Build history of the part. All positions in model axes, mm. Round coordinates to 2 decimals unless told otherwise and drop trailing zeros. Order: outer loops, then holes, each group sorted by start corner. A loop starts at its lowest first (then second) coordinate and runs counter-clockwise, first axis right, second up. Notation, with made-up numbers: M 65.5,85 L 75.5,85 A21 ccw 75.5,117 Z; hole C 80,-0.5 d2. An arc over 180 degrees is marked long. Use CSV: the item, a comma, the result in double quotes.
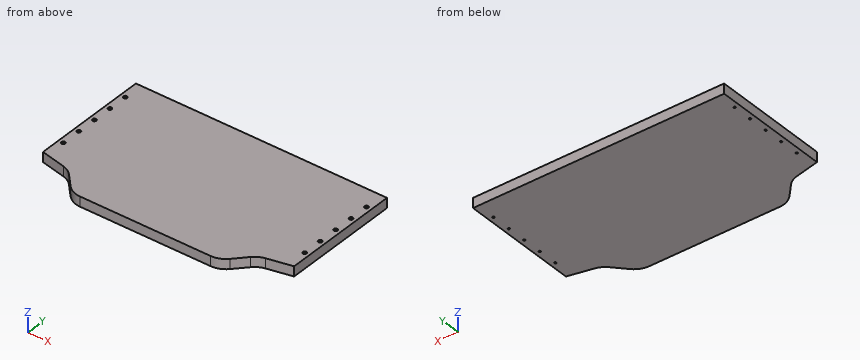
from build123d import *

# Parameters (mm, degrees)
BOSS_EXTRUDE1_DEPTH                        = 25.4
FILLET1_R                                  = 50.8
CSK_FOR_10_FLAT_HEAD_MACHINE_SCREW_2_COUNT = 2
CSK_FOR_10_FLAT_HEAD_MACHINE_SCREW_2_PITCH = 50.8
CSK_FOR_10_FLAT_HEAD_MACHINE_SCREW_3_COUNT = 2
CSK_FOR_10_FLAT_HEAD_MACHINE_SCREW_3_PITCH = 101.6
CSK_FOR_10_FLAT_HEAD_MACHINE_SCREW_4_COUNT = 2
CSK_FOR_10_FLAT_HEAD_MACHINE_SCREW_4_PITCH = 152.4
CSK_FOR_10_FLAT_HEAD_MACHINE_SCREW_5_COUNT = 2
CSK_FOR_10_FLAT_HEAD_MACHINE_SCREW_5_PITCH = 203.2


with BuildPart() as part:
    # Sketch1 → Boss-Extrude1 (new body)
    with BuildSketch(Plane.XY):
        Polygon((-245.162116144, 59.122546749), (-190.5, 0), (190.5, 0), (245.162116144, 59.122546749), (323.85, 76.2), (323.85, 381), (-323.85, 381), (-323.85, 76.2), align=None)
    extrude(amount=BOSS_EXTRUDE1_DEPTH)

    # Fillet1
    fillet1_edges = [part.edges().sort_by_distance(p)[0] for p in [
        (245.162116144, 59.122546749, 12.7),
        (190.5, 0, 12.7),
        (-190.5, 0, 12.7),
        (-245.162116144, 59.122546749, 12.7),
    ]]
    fillet(fillet1_edges, radius=FILLET1_R)

    # Sketch4 → CSK for #10 Flat Head Machine Screw (100)1 (revolve, cut)
    with BuildSketch(Plane(origin=(311.15, 330.2, 25.4), x_dir=(0, -1, 0), z_dir=(1, 0, 0))):
        Polygon((0, 0), (0, 52.333816902), (2.5527, 50.8), (2.5527, 1.960808018), (4.8895, 0), align=None)
    csk_for_10_flat_head_machine_screw_100 = revolve(axis=Axis((311.15, 330.2, 31.75), (0, 0, -1)), mode=Mode.SUBTRACT)

    # CSK for _10 Flat Head Machine Screw  2: CSK for #10 Flat Head Machine Screw (100)1 ×2
    with Locations(*[(0, -i * CSK_FOR_10_FLAT_HEAD_MACHINE_SCREW_2_PITCH, 0) for i in range(1, CSK_FOR_10_FLAT_HEAD_MACHINE_SCREW_2_COUNT)]):
        add(csk_for_10_flat_head_machine_screw_100, mode=Mode.SUBTRACT)

    # CSK for _10 Flat Head Machine Screw  3: CSK for #10 Flat Head Machine Screw (100)1 ×2
    with Locations(*[(0, -i * CSK_FOR_10_FLAT_HEAD_MACHINE_SCREW_3_PITCH, 0) for i in range(1, CSK_FOR_10_FLAT_HEAD_MACHINE_SCREW_3_COUNT)]):
        add(csk_for_10_flat_head_machine_screw_100, mode=Mode.SUBTRACT)

    # CSK for _10 Flat Head Machine Screw  4: CSK for #10 Flat Head Machine Screw (100)1 ×2
    with Locations(*[(0, -i * CSK_FOR_10_FLAT_HEAD_MACHINE_SCREW_4_PITCH, 0) for i in range(1, CSK_FOR_10_FLAT_HEAD_MACHINE_SCREW_4_COUNT)]):
        add(csk_for_10_flat_head_machine_screw_100, mode=Mode.SUBTRACT)

    # CSK for _10 Flat Head Machine Screw  5: CSK for #10 Flat Head Machine Screw (100)1 ×2
    with Locations(*[(0, -i * CSK_FOR_10_FLAT_HEAD_MACHINE_SCREW_5_PITCH, 0) for i in range(1, CSK_FOR_10_FLAT_HEAD_MACHINE_SCREW_5_COUNT)]):
        add(csk_for_10_flat_head_machine_screw_100, mode=Mode.SUBTRACT)

    # Mirror1: CSK for #10 Flat Head Machine Screw (100)1 across plane
    add(csk_for_10_flat_head_machine_screw_100.mirror(Plane(origin=(0, 0, 0), x_dir=(0, 0, 1), z_dir=(1, 0, 0))), mode=Mode.SUBTRACT)

    # Mirror1 copy 1 sketch → Mirror1 copy 1 (revolve, cut)
    with BuildSketch(Plane(origin=(-311.15, 279.4, 25.4), x_dir=(0, -1, 0), z_dir=(-1, 0, 0))):
        Polygon((0, 0), (0, -52.333816902), (2.5527, -50.8), (2.5527, -1.960808018), (4.8895, 0), align=None)
    revolve(axis=Axis((-311.15, 279.4, 31.75), (0, 0, 1)), mode=Mode.SUBTRACT)

    # Mirror1 copy 2 sketch → Mirror1 copy 2 (revolve, cut)
    with BuildSketch(Plane(origin=(-311.15, 228.6, 25.4), x_dir=(0, -1, 0), z_dir=(-1, 0, 0))):
        Polygon((0, 0), (0, -52.333816902), (2.5527, -50.8), (2.5527, -1.960808018), (4.8895, 0), align=None)
    revolve(axis=Axis((-311.15, 228.6, 31.75), (0, 0, 1)), mode=Mode.SUBTRACT)

    # Mirror1 copy 3 sketch → Mirror1 copy 3 (revolve, cut)
    with BuildSketch(Plane(origin=(-311.15, 177.8, 25.4), x_dir=(0, -1, 0), z_dir=(-1, 0, 0))):
        Polygon((0, 0), (0, -52.333816902), (2.5527, -50.8), (2.5527, -1.960808018), (4.8895, 0), align=None)
    revolve(axis=Axis((-311.15, 177.8, 31.75), (0, 0, 1)), mode=Mode.SUBTRACT)

    # Mirror1 copy 4 sketch → Mirror1 copy 4 (revolve, cut)
    with BuildSketch(Plane(origin=(-311.15, 127, 25.4), x_dir=(0, -1, 0), z_dir=(-1, 0, 0))):
        Polygon((0, 0), (0, -52.333816902), (2.5527, -50.8), (2.5527, -1.960808018), (4.8895, 0), align=None)
    revolve(axis=Axis((-311.15, 127, 31.75), (0, 0, 1)), mode=Mode.SUBTRACT)


solid = part.part
(1) Cut at A-A, the plane z = 16. Count the separate pieces of the cut face and the enclosed holes in it, and give its area (3 significant figures).
Answer block:
separate pieces,"1"
enclosed holes,"10"
area,"233,000 mm²"
(2) Cut at B-B, the plane x = 272. Give the cut face in (y, z).
Answer block:
outline,"M 64.95,0 L 381,0 L 381,25.4 L 64.95,25.4 Z"
(3) Drop flat-ended pins along their axis: pin 1 (4 mm diameter, centred on x = -311.15, y = 177.8, fed in from -Z); pin 2 (10 mm diameter, centred on x = 201.5, z = 3, fed in from -Y); pin 3 (8 mm diameter, centred on x = 311.15, y = 127, fed in from +Z). Give the stop position or say it passes through.
Answer block:
pin 1,"passes through"
pin 2,"stops at y = 8.56"
pin 3,"stops at z = 24.65"
(4) Wall check: line 1 (X direction, y = 228.6, z = 18.75); line 2 (Y direction, x = 311.15, z = 5); line 3 (Y direction, x = -259, z = 7). Give the ranges that are in metal, low to high. Write a range as from..to.
Answer block:
line 1,"x = -323.85..-313.7, -308.6..308.6, 313.7..323.85"
line 2,"y = 73.44..124.45, 129.55..175.25, 180.35..226.05, 231.15..276.85, 281.95..327.65, 332.75..381"
line 3,"y = 62.09..381"
